The model under review builds one solid part; all positions refer to its coordinate system, in mm. A direction names the side the tool comes from. Coordinates: 2 decimals unless noted, no trailing zeros. Write each loop counter-clockwise with the first axis right and the second up, starting at its lowest first coordinate (ties: lowest second). Pieces come first, ordered by that corner, then holes. Notation, with made-up numbers: (13.25, 84.25) - (51.25, 84.25) arc R17 ccw to (51.25, 104.25) - close; hole circle Ø3 at (38.25, 77.5). An arc over 180 degrees is marked (long way). Use one line per item in the form item = value. Start each with the question number.
```python
from build123d import *

# Parameters (mm, degrees)
F1_DEPTH = 10
F2_R     = 3
F3_SIZE  = 1


with BuildPart() as f1:
    # F0 (on Top) → F1 (new body)
    with BuildSketch(Plane.XY):
        Polygon((0, 14.626703), (0, 7.313351), (3, 7.313351), (7.313351, 11.626703), (7.313351, 14.626703), align=None)
        Polygon((0, 7.313351), (0, 0), (7.313351, 0), (7.313351, 3), (3, 7.313351), align=None)
        Polygon((7.313351, 3), (7.313351, 0), (14.626703, 0), (14.626703, 7.313351), (11.626703, 7.313351), align=None)
        Polygon((11.626703, 7.313351), (14.626703, 7.313351), (14.626703, 14.626703), (7.313351, 14.626703), (7.313351, 11.626703), align=None)
    extrude(amount=F1_DEPTH)

    # F2
    f2_edges = [f1.edges().sort_by_distance(p)[0] for p in [
        (0, 0, 5),
        (0, 14.626703, 5),
        (14.626703, 0, 5),
        (14.626703, 14.626703, 5),
    ]]
    fillet(f2_edges, radius=F2_R)

    # F3
    f3_edges = [f1.edges().sort_by_distance(p)[0] for p in [
        (5.156676, 9.470027, 10),
        (5.156676, 5.156676, 10),
        (9.470027, 9.470027, 10),
        (9.470027, 5.156676, 10),
    ]]
    chamfer(f3_edges, length=F3_SIZE)


solid = f1.part
```
1. Take a section at A-A (y = 9.75). State the section outline as (x, z) points.
2. Take a section at B-B (x = 4). State the section outline as (y, z) points, plus the area to 3 significant figures.
3. For L1, parallel to X at y = 3.5, z = 6.25; L2, parallel to X at y = 6.5, z = 4.25; L3, parallel to Y at x = 5, z = 7, list the stretches that pass through material, from the lowest coordinate up.
4. For faces 5 (the cylindrical face through (13.725, 0.855, 5.07)), 6 (the flat face through (5.187, 5.126, 4.437)), 7 (the flat face through (4.77, 9.78, 9.49)), list the 3-axis set-ups (+Z, -Z, +X, -X, +Y, -Y) from which the entire face can be reached by the end or side of a thin tool; tool diameter is ignored.
5. Take a section at C-C (z = 8.25). State the section outline as (x, y) points, plus the area to 3 significant figures.
6. Take a section at D-D (y = 13.5). State the section outline as (x, z) points, plus the area to 3 significant figures.
7. The part is to be moulded in two halves that separate along X. For faces 1 (the flat face through (0, 7, 5)), 2 (the flat face through (9.779, 9.859, 9.493)), 3 (the cylindrical face through (13.771, 13.725, 5.07)), 4 (the flat face through (4.85, 4.77, 9.49)), say which applies: released by +X, released by -X, zero draft, split by the parting line, or undercut.
Returned:
q1.outline = (0, 0) - (5.44, 0) - (5.44, 9) - (4.02, 10) - (0, 10) - close; (9.19, 0) - (14.63, 0) - (14.63, 10) - (10.6, 10) - (9.19, 9) - close
q2.outline = (0, 0) - (6.31, 0) - (6.31, 9) - (4.9, 10) - (0, 10) - close; (8.31, 0) - (14.63, 0) - (14.63, 10) - (9.73, 10) - (8.31, 9) - close
q2.area = 125 mm²
q3.L1 = 0 to 6.81, 7.81 to 14.63
q3.L2 = 0 to 3.81, 10.81 to 14.63
q3.L3 = 0 to 5.31, 9.31 to 14.63
q4.face_5 = +Z, -Z, +X, -Y
q4.face_6 = +Z, -Z
q4.face_7 = +Z
q5.outline = (0, 3) arc R3 ccw to (3, 0) - (11.63, 0) arc R3 ccw to (14.63, 3) - (14.63, 11.63) arc R3 ccw to (11.63, 14.63) - (3, 14.63) arc R3 ccw to (0, 11.63) - close; hole (3, 7.31) - (7.31, 3) - (11.63, 7.31) - (7.31, 11.63) - close
q5.area = 169 mm²
q6.outline = (0.66, 0) - (13.97, 0) - (13.97, 10) - (0.66, 10) - close
q6.area = 133 mm²
q7.face_1 = released by -X
q7.face_2 = undercut
q7.face_3 = released by +X
q7.face_4 = undercut
